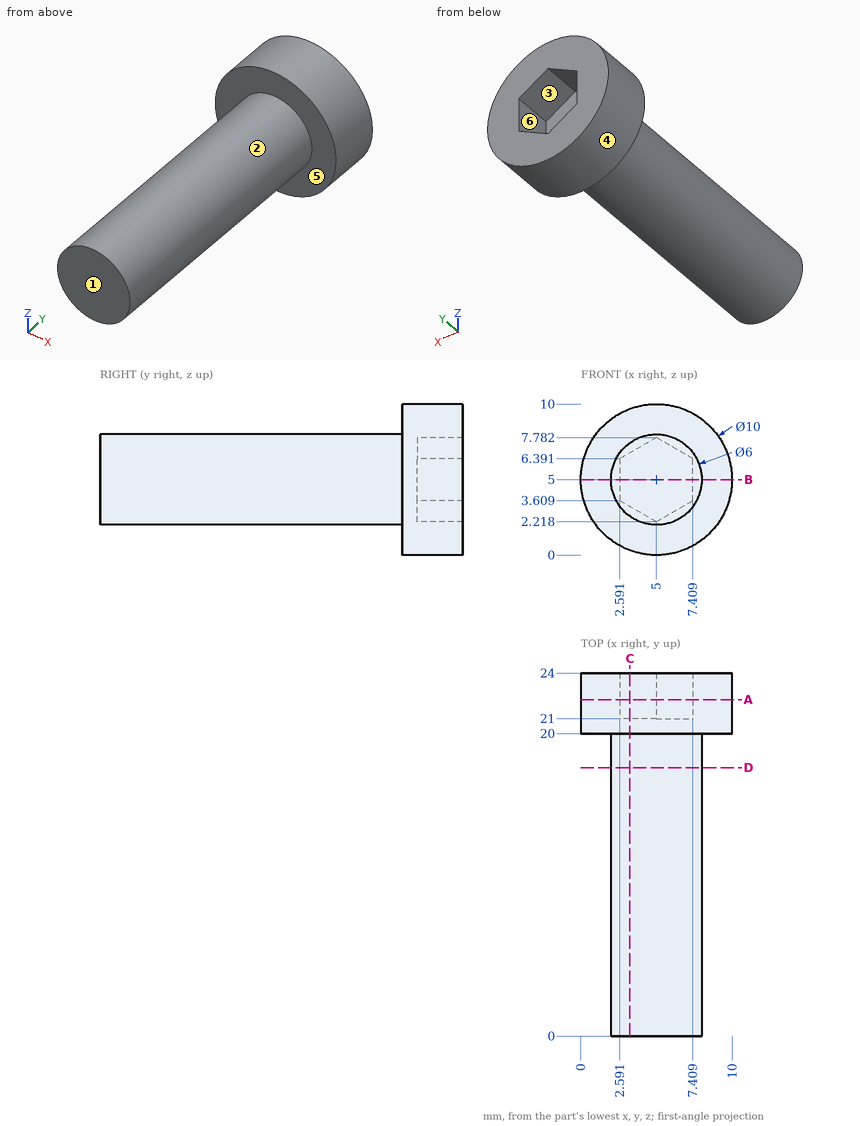
Check sheet for the drawn part. Datum: minimum x, y, z corner. Units: mm. A direction names the side the tool comes from. Give positions to 0.01 mm unless a question says otherwise; leave off trailing zeros. Write each loop counter-clockwise with the first axis right and the second up, starting at its lowest first coordinate (ties: lowest second). Pieces come first, ordered by that corner, then holes.
(1) Cross-section at A-A (y = 22.25). Enter the section's corners in (x, z).
(2) Cross-section at B-B (z = 5). Enter the section's corners in (x, y).
(3) Material ranges on line 1 (Y direction, x = 5.25, z = 3.25); line 2 (Z direction, x = 1, y = 20.5); line 3 (Y direction, x = 1, z = 6.75), recorded low to high.
(4) Access from +Z, -Z, +X, -X, +Y, -Y to the whole of each face (thin tool, end or side, straight path). Record for the marked faces 1, 2 and 3.
(5) Gauge pin test, flat ends, axial feed: pin 1 (1.4 mm diameter, centred on x = 6, z = 4.5, fed in from +Y); pin 2 (5 mm diameter, centred on y = 12, z = 4, fed in from -X). Record the tip position at first contact, or that the pin passes through.
(6) Cross-section at D-D (y = 17.75). Enter the section's corners in (x, z).
(7) Mould release check, pull along Z, two halves, no side actions. Record for the marked faces 4, 5 and 6: +Z half, -Z half, draft (parallel to the pull), parting line (faces both ways), or undercut.
(8) Cross-section at C-C (x = 3.25). Enter the section's corners in (y, z).
Worked out:
1. outline: circle Ø10 at (5, 5); hole (2.59, 3.61) - (5, 2.22) - (7.41, 3.61) - (7.41, 6.39) - (5, 7.78) - (2.59, 6.39) - close
2. outline: (0, 20) - (2, 20) - (2, 0) - (8, 0) - (8, 20) - (10, 20) - (10, 24) - (7.41, 24) - (7.41, 21) - (2.59, 21) - (2.59, 24) - (0, 24) - close
3. line 1: y = 0 to 21
3. line 2: z = 2 to 8
3. line 3: y = 20 to 24
4. face 1: +Z, -Z, +X, -X, -Y
4. face 2: -Y
4. face 3: +Y
5. pin 1: stops at y = 21
5. pin 2: stops at x = 2
6. outline: circle Ø6 at (5, 5)
7. face 4: parting line
7. face 5: draft
7. face 6: undercut
8. outline: (0, 2.56) - (20, 2.56) - (20, 0.32) - (24, 0.32) - (24, 3.23) - (21, 3.23) - (21, 6.77) - (24, 6.77) - (24, 9.68) - (20, 9.68) - (20, 7.44) - (0, 7.44) - close
